from build123d import *

# Parameters (mm, degrees)
F0_W     = 500
F0_H     = 500
F1_DEPTH = 15
F2_W     = 20
F2_H     = 100
F3_DEPTH = 110
F4_R     = 15
F5_DEPTH = 490.001


with BuildPart() as f1:
    # F0 (on Top) → F1 (new body)
    with BuildSketch(Plane.XY):
        Rectangle(F0_W, F0_H)
    extrude(amount=F1_DEPTH)

    # F2 (on face) → F3 (join)
    with BuildSketch(Plane.XY.offset(15)):
        with Locations((230, 200)):
            Rectangle(F2_W, F2_H)
        with Locations((-230, 200)):
            Rectangle(F2_W, F2_H)
    extrude(amount=F3_DEPTH)

    # F4 (on face) → F5 (cut, through all)
    with BuildSketch(Plane.YZ.offset(240)):
        with Locations((200, 85)):
            Circle(F4_R)
    extrude(amount=-F5_DEPTH, mode=Mode.SUBTRACT)


solid = f1.part
CAD build for the part. Positions are in the model's coordinates, mm. A direction names the side the tool comes from. Coordinates: 2 decimals unless noted, no trailing zeros. Write each loop counter-clockwise with the first axis right and the second up, starting at its lowest first coordinate (ties: lowest second). Pieces come first, ordered by that corner, then holes. Notation, with made-up numbers: M -32,-1.5 L -16,-1.5 A21 cw -16,17.5 Z; hole C -3.5,23 d7. An arc over 180 degrees is marked long. Return JSON: item names as keys, results as strings.
Item 1: Slice it at A-A, the plane z = 85. Write the cut outline in (x, y).
Findings below:
{"outline": "M -240,150 L -220,150 L -220,185 L -240,185 Z; M -240,215 L -220,215 L -220,250 L -240,250 Z; M 220,150 L 240,150 L 240,185 L 220,185 Z; M 220,215 L 240,215 L 240,250 L 220,250 Z"}
Item 2: Probe line 1 (X direction, y = 167, z = 29); line 2 (Z direction, x = 233, y = 200); line 3 (Z direction, x = 162, y = -4.5). List the from-to ranges inside material, lowest first. Write a range as from..to.
Findings below:
{"line 1": "x = -240..-220, 220..240", "line 2": "z = 0..70, 100..125", "line 3": "z = 0..15"}
Item 3: Two-plate mould, pull along Y, no slides. Class faces 1 (the flat face through (-3, -250, 7)), 2 (the cylindrical face through (230.14, 196.748, 70.357)), 3 (the cylindrical face through (-229.86, 196.748, 70.357)), 4 (the flat face through (220, 199, 69)): +Y half, -Y half, draft (parallel to the pull), parting line (faces both ways), or undercut.
Findings below:
{"face 1": "-Y half", "face 2": "undercut", "face 3": "undercut", "face 4": "draft"}
Item 4: Drop flat-ended pins along their axis: pin 1 Ø18 at (y, z) = (200, 85) entering from +X; pin 2 Ø5 at (x, y) = (-16, 54.5) entering from +Z; pin 3 Ø22 at (x, z) = (-231.5, 72.5) entering from -Y. Give the stop position or say it passes through.
Findings below:
{"pin 1": "passes through", "pin 2": "stops at z = 15", "pin 3": "stops at y = 150"}
Item 5: Which spindle directions (+Z, -Z, +X, -X, +Y, -Y) get a long thin tool onto all of the face, cutting with end or side? Do faces 5 (the flat face through (-220, 199, 69)), 6 (the flat face through (-230, 150, 69)), 7 (the flat face through (240, 199, 69)), 8 (the flat face through (-240, 199, 69)). Say none if no direction does.
Findings below:
{"face 5": "+Z, +Y, -Y", "face 6": "+Z, +X, -X, -Y", "face 7": "+Z, +X, +Y, -Y", "face 8": "+Z, -X, +Y, -Y"}
Item 6: Slice it at B-B, the plane y = 200. Write the cut outline in (x, z).
Findings below:
{"outline": "M -250,0 L 250,0 L 250,15 L 240,15 L 240,70 L 220,70 L 220,15 L -220,15 L -220,70 L -240,70 L -240,15 L -250,15 Z; M -240,100 L -220,100 L -220,125 L -240,125 Z; M 220,100 L 240,100 L 240,125 L 220,125 Z"}
Item 7: Slice it at C-C, the plane x = 151. Write the cut outline in (y, z).
Findings below:
{"outline": "M -250,0 L 250,0 L 250,15 L -250,15 Z"}
